The listing builds one solid part. Answer for the finished solid, in the listing's coordinates (mm). Face numbers are marked on the shaded views. A direction names the side the tool comes from. Give positions to 0.01 mm unless a question says otherwise; leave off trailing zeros. Order: outer loops, then holes, each group sorted by start corner. A loop starts at its lowest first (then second) coordinate and runs counter-clockwise, first axis right, second up. Notation, with made-up numbers: (-22, -27.75) - (-15, -27.75) arc R32 ccw to (-15, -0.75) - close; hole circle Ø6 at (38, -32.5). An arc over 180 degrees is marked (long way). Answer as CSV lines item,"result". Start each with the question number.
1. Section A-A on x = 4 is taken. Give the vertices of the cut face in (y, z).
2. Flat-ended cylindrical pins translate along their axes: pin 1 (5.5 mm diameter, centred on x = 11.5, y = 5, fed in from -Z); pin 2 (3 mm diameter, centred on x = 24.5, y = 6, fed in from +Z); pin 3 (5 mm diameter, centred on x = 10, z = 10, fed in from -Y); pin 4 (0.9 mm diameter, centred on y = 1, z = 34.5, fed in from +X). Find the tip coordinate at first contact, or state that the pin passes through.
3. Consider line 1 along Z through (x, y) = (10, 7.55); line 2 along Z through (x, y) = (10, 2.75); line 3 along X through (y, z) = (3.1, 25). Determine where each line is inside the solid, lowest interval first. Write a range as [from, to].
4. Section D-D on z = 25 is taken. Give the vertices of the cut face in (x, y), and give its area (3 significant figures).
5. Section C-C on y = 1.75 is taken. Give the vertices of the cut face in (x, z).
6. Which of the six approach directions +Z, -Z, +X, -X, +Y, -Y give full straight-line access (tool end or side, diameter ignored) to the marked faces 4 and 5?
7. Section B-B on z = 45.5 is taken. Give the vertices of the cut face in (x, y).
8. Determine the mould class of the marked faces 1, 2 and 3 for opening direction X: +X half, -X half, draft (parallel to the pull), parting line (faces both ways), or undercut.
from build123d import *

# Parameters (mm, degrees)
F0_R     = 1.3
F0_R_2   = 1.85
F0_R_3   = 1.5
F1_DEPTH = 3
F2_DEPTH = 10
F3_D     = 6
F3_DEPTH = 5
F3_TIP   = 1.8025818571


with BuildPart() as f1:
    # F0 (on Front) → F1 (new body)
    with BuildSketch(Plane.XZ):
        Polygon((-10.5, -5), (51.5, -5), (51.5, 12.5), (14, 12.5), (14, 6), (6, 6), (6, 29), (8, 29), (8, 49.5), (0, 49.5), (0, 3), (-10.5, 3), align=None)
        with Locations((-6.5, -1)):
            Circle(F0_R, mode=Mode.SUBTRACT)
        with Locations((26.5, -1)):
            Circle(F0_R, mode=Mode.SUBTRACT)
        with Locations((47.5, 8.5)):
            Circle(F0_R_2, mode=Mode.SUBTRACT)
        with Locations((4, 45.5)):
            Circle(F0_R_2, mode=Mode.SUBTRACT)
        Polygon((14, 6), (14, 12.5), (14, 29), (8, 29), (6, 29), (6, 6), align=None)
        with Locations((10, 10)):
            Circle(F0_R_3, mode=Mode.SUBTRACT)
        with Locations((10, 25)):
            Circle(F0_R_3, mode=Mode.SUBTRACT)
    extrude(amount=-F1_DEPTH)

    # F0 (on Front) → F2 (join)
    with BuildSketch(Plane.XZ):
        Polygon((14, 6), (14, 12.5), (14, 29), (8, 29), (6, 29), (6, 6), align=None)
        with Locations((10, 10)):
            Circle(F0_R_3, mode=Mode.SUBTRACT)
        with Locations((10, 25)):
            Circle(F0_R_3, mode=Mode.SUBTRACT)
    extrude(amount=-F2_DEPTH)

    # F3
    with Locations(Plane.XZ):
        with Locations((10, 25), (10, 10)):
            Hole(F3_D / 2, depth=F3_DEPTH)
            with Locations((0, 0, -(F3_DEPTH + F3_TIP / 2))):  # 118° drill point
                Cone(0, F3_D / 2, F3_TIP, mode=Mode.SUBTRACT)


solid = f1.part
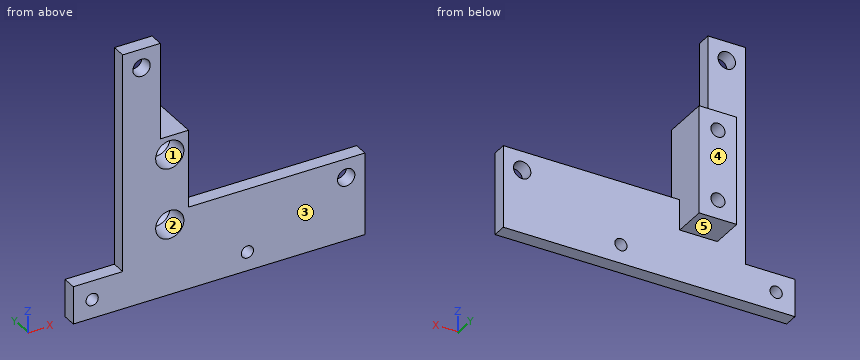
Checks:
1,outline,"(0, -5) - (3, -5) - (3, 43.65) - (0, 43.65) - close; (0, 47.35) - (3, 47.35) - (3, 49.5) - (0, 49.5) - close"
2,pin 1,"stops at z = -5"
2,pin 2,"passes through"
2,pin 3,"stops at y = 5.3"
2,pin 4,"stops at x = 8"
3,line 1,"z = [6, 8.5], [11.5, 23.5], [26.5, 29]"
3,line 2,"z = [-5, 7], [13, 22], [28, 29]"
3,line 3,"x = [6, 7], [13, 14]"
4,outline,"(0, 0) - (7, 0) - (7, 5) - (8.5, 5.9) - (8.5, 10) - (6, 10) - (6, 3) - (0, 3) - close; (11.5, 5.9) - (13, 5) - (13, 0) - (14, 0) - (14, 10) - (11.5, 10) - close"
4,area,"51.6 mm²"
5,outline,"(-10.5, -5) - (51.5, -5) - (51.5, 12.5) - (14, 12.5) - (14, 29) - (8, 29) - (8, 49.5) - (0, 49.5) - (0, 3) - (-10.5, 3) - close; hole circle Ø2.6 at (-6.5, -1); hole circle Ø3.7 at (4, 45.5); hole circle Ø6 at (10, 10); hole circle Ø6 at (10, 25); hole circle Ø2.6 at (26.5, -1); hole circle Ø3.7 at (47.5, 8.5)"
6,face 4,"+Z, -Z, +X, -X, +Y"
6,face 5,"-Z, +X, -X, +Y"
7,outline,"(0, 0) - (2.15, 0) - (2.15, 3) - (0, 3) - close; (5.85, 0) - (8, 0) - (8, 3) - (5.85, 3) - close"
8,face 1,"undercut"
8,face 2,"undercut"
8,face 3,"draft"
